```python
from build123d import *

# Parameters (mm, degrees)
F0_W     = 32
F0_H     = 32
F0_R     = 0.6
F0_R_2   = 14.5
F1_DEPTH = 2
F2_R     = 8
F3_SIZE  = 1


with BuildPart() as f1:
    # F0 (on Top) → F1 (new body)
    with BuildSketch(Plane.XY):
        with Locations((16, -16)):
            Rectangle(F0_W, F0_H)
        with Locations((4, -28)):
            Circle(F0_R, mode=Mode.SUBTRACT)
        with BuildLine():
            ThreePointArc((28.6, -28), (28.5543277195, -28.2296100594), (28.4242640687, -28.4242640687))
            ThreePointArc((28.4242640687, -28.4242640687), (27.4456722805, -27.7703899406), (28.6, -28))
        make_face(mode=Mode.SUBTRACT)
        with BuildLine():
            ThreePointArc((4.6, -4), (3.7703899406, -4.5543277195), (3.5757359313, -3.5757359313))
            ThreePointArc((3.5757359313, -3.5757359313), (4.2296100594, -3.4456722805), (4.6, -4))
        make_face(mode=Mode.SUBTRACT)
        with Locations((16, -16)):
            Circle(F0_R_2, mode=Mode.SUBTRACT)
        with Locations((28, -4)):
            Circle(F0_R, mode=Mode.SUBTRACT)
    extrude(amount=F1_DEPTH)

    # F2
    f2_edges = [f1.edges().sort_by_distance(p)[0] for p in [
        (32, 0, 1),
        (0, 0, 1),
        (0, -32, 1),
        (32, -32, 1),
    ]]
    fillet(f2_edges, radius=F2_R)

    # F3
    f3_edges = [f1.edges().sort_by_distance(p)[0] for p in [
        (2.343146, -2.343146, 2),
    ]]
    chamfer(f3_edges, length=F3_SIZE)


solid = f1.part
```
Here's how the part is built. I have some questions about the finished solid (model axes, mm). Round coordinates to 2 decimals unless told otherwise and drop trailing zeros. Loops run counter-clockwise (first coordinate to the right, second up) from the corner with the lowest first, then second, coordinate; pieces in that order, holes last.
1. Thinking about a two-plate mould opening in X: for faces 1 (the face through (4.49, -24.82, 0.99)), 2 (the face through (3.922, -27.405, 0.986)), 3 (the face through (2.281, -2.406, 0.507)), 4 (the face through (16.1, -31.5, 1.5)), which applies, released by +X, released by -X, zero draft, split by the parting line, or undercut?
Answers:
face 1: undercut
face 2: undercut
face 3: released by -X
face 4: zero draft
2. Suppose I cut it at C-C, the plane x = 28. Give the number of separate pieces and of enclosed holes in the cut face, and give its area (3 significant figures).
Answers:
separate pieces: 4
enclosed holes: 0
area: 21.2 mm2
3. Suppose I cut it at B-B, the plane y = -9. Please give me the cut outline in (x, z).
Answers:
outline: (0, 0) - (3.3, 0) - (3.3, 2) - (1, 2) - (0, 1) - close; (28.7, 0) - (32, 0) - (32, 1) - (31, 2) - (28.7, 2) - close
4. If I drill on probe 1 along X at (y, z) = (-3.5, 1.6); probe 2 along Y at (x, z) = (28, 1.1); probe 3 along Y at (x, z) = (4, 1.25), over which ranges is the centre line in solid material (lowest first)?
Answers:
probe 1: x = 2.13 to 3.67, 4.33 to 8.65, 23.35 to 27.67, 28.33 to 29.87
probe 2: y = -30.81 to -28.6, -27.4 to -24.14, -7.86 to -4.6, -3.4 to -1.19
probe 3: y = -30.64 to -28.6, -27.4 to -24.14, -7.86 to -4.6, -3.4 to -1.36
5. Suppose I cut it at A-A, the plane x = 16. Please give me the cut outline in (y, z), and give its area (3 significant figures).
Answers:
outline: (-32, 0) - (-30.5, 0) - (-30.5, 2) - (-31, 2) - (-32, 1) - close; (-1.5, 0) - (0, 0) - (0, 1) - (-1, 2) - (-1.5, 2) - close
area: 5.00 mm2
6. Will this pin go through, and if not, where does the flat tip stop? pin 1 (6 mm diameter, centred on x = 9.5, y = -8, fed in from -Z).
Answers:
pin 1: passes through
